Answer from the drawing. Dimensions are ordinates in mm from the lowest x, y and z of the part. A direction names the side the tool comes from. Give positions to 0.01 mm unless a question says otherwise; leave off trailing zeros. Order: outer loops, then holes, each group sorted by start corner. A loop starts at its lowest first (then second) coordinate and runs counter-clockwise, first axis right, second up. Notation, with made-up numbers: (-19.5, 10.5) - (14.5, 10.5) arc R31 cw to (14.5, 49.5) - close; hole circle Ø5 at (52, -1). An arc over 180 degrees is marked (long way). Write each question's results on one line, items separated by ' | '.
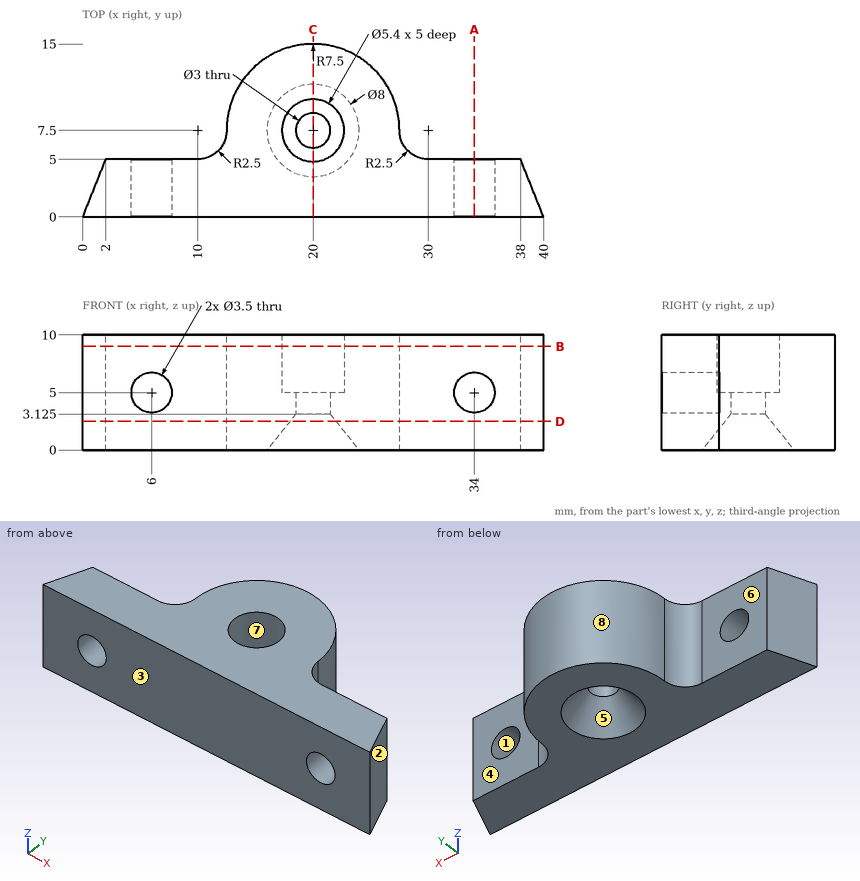
1. A cutting plane is placed at D-D, the plane z = 2.5. Write down the section's boundary in (x, y), then the cut area to 3 significant figures.
Answer list:
outline: (0, 0) - (40, 0) - (38, 5) - (30, 5) arc R2.5 cw to (27.5, 7.5) arc R7.5 ccw to (12.5, 7.5) arc R2.5 cw to (10, 5) - (2, 5) - close; hole circle Ø4 at (20, 7.5) | area: 306 mm^2
2. Straight lines are drawn through the part: line 1 (Y direction, x = 20, z = 6.65); line 2 (X direction, y = 2.65, z = 5); line 3 (X direction, y = 1, z = 4.25). For each, find the intervals that lie inside material, in ascending order. Write a range as [from, to].
Answer list:
line 1: [0, 4.8], [10.2, 15] | line 2: [1.06, 4.25], [7.75, 32.25], [35.75, 38.94] | line 3: [0.4, 4.42], [7.58, 32.42], [35.58, 39.6]
3. A cutting plane is placed at C-C, the plane x = 20. Write down the section's boundary in (y, z) (3 decimals).
Answer list:
outline: (0, 0) - (3.5, 0) - (6, 3.125) - (6, 5) - (4.8, 5) - (4.8, 10) - (0, 10) - close; (9, 3.125) - (11.5, 0) - (15, 0) - (15, 10) - (10.2, 10) - (10.2, 5) - (9, 5) - close
4. A cutting plane is placed at B-B, the plane z = 9. Write down the section's boundary in (x, y), then the cut area to 3 significant figures.
Answer list:
outline: (0, 0) - (40, 0) - (38, 5) - (30, 5) arc R2.5 cw to (27.5, 7.5) arc R7.5 ccw to (12.5, 7.5) arc R2.5 cw to (10, 5) - (2, 5) - close; hole circle Ø5.4 at (20, 7.5) | area: 296 mm^2
5. A cutting plane is placed at A-A, the plane x = 34. Write down the section's boundary in (y, z).
Answer list:
outline: (0, 0) - (5, 0) - (5, 3.25) - (0, 3.25) - close; (0, 6.75) - (5, 6.75) - (5, 10) - (0, 10) - close
6. A tool of negligible diameter and unlimited length cuts with its end or side. For the marked faces 4, 5, 6, 7 and 8, from which of +Z, -Z, +X, -X, +Y, -Y can it reach the whole face along a straight path? Write none if from no direction.
Answer list:
face 4: +Z, -Z, +X, +Y | face 5: -Z | face 6: +Z, -Z, -X, +Y | face 7: +Z | face 8: +Z, -Z, +Y
7. Determine the mould class of the marked faces 1, 2 and 3 for opening direction X: +X half, -X half, draft (parallel to the pull), parting line (faces both ways), or undercut.
Answer list:
face 1: undercut | face 2: +X half | face 3: draft
8. Given P1, Ø4, axis at x = 6, z = 5, coming from the +Y side; P2, Ø3, axis at y = 3, z = 4, coming from the +X side; P3, Ø5, axis at x = 20, y = 7.5, coming from the -Z side (3 decimals), each flat-ended and moving along its own axis, determine where each tip first touches the part or whether it passes through.
Answer list:
P1: y = 5 | P2: x = 39.4 | P3: z = 1.875
